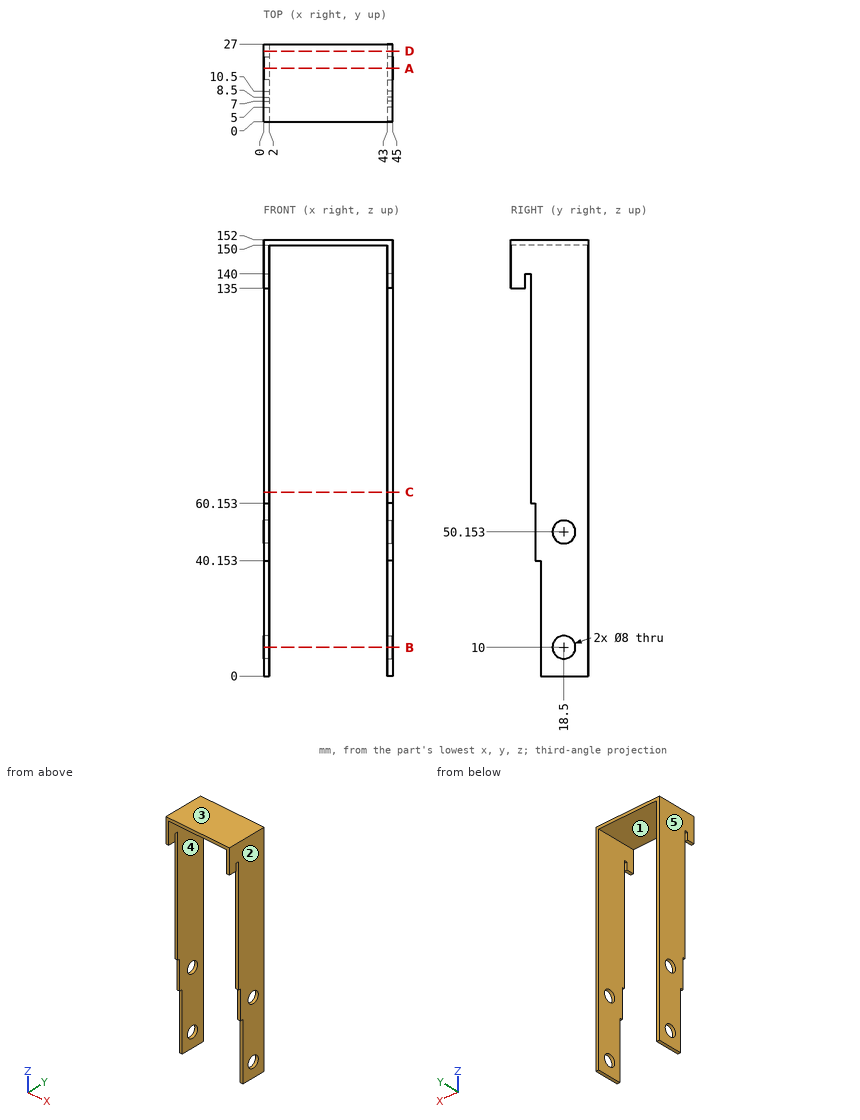
Source: three-view drawing plus pictorial views. Frame: mm from the lowest corner of the part. A direction names the side the tool comes from. Round coordinates to 2 decimals unless told otherwise and drop trailing zeros. Loops run counter-clockwise (first coordinate to the right, second up) from the corner with the lowest first, then second, coordinate; pieces in that order, holes last. Notation, with made-up numbers: (-7, -33) - (-2, -33) arc R25 cw to (-2, -19) - close; hole circle Ø8 at (77.25, 22.25). An arc over 180 degrees is marked (long way). Write item = value, one per line. Start each with the question number.
Item 1: Reachability of the marked faces 4 and 5 from +Z, -Z, +X, -X, +Y, -Y: full face, straight path, thin tool, end or side. Return the list, or none.
Item 2: First-contact query: pin 1 Ø1.5 at (y, z) = (8, 103.5) entering from -X; pin 2 Ø0.6 at (x, y) = (1, 10) entering from -Z; pin 3 Ø0.6 at (x, y) = (44, 1.5) entering from -Z; pin 4 Ø3 at (x, y) = (17, 19.5) entering from -Z. Flat tips, straight axial feed; report the tip coordinate or a pass-through.
Item 3: Mould query, pull axis X, two halves, no side actions, for the marked faces 1, 2 and 3. Classes: released by +X, released by -X, zero draft, split by the parting line, or undercut.
Item 4: Material intervals for line 1 (Z direction, x = 0.5, y = 18.5); line 2 (X direction, y = 23, z = 145); line 3 (Z direction, x = 29, y = 16.5), sorted ascending.
Item 5: Section query D-D on y = 24.5. Output: boundary loops of the cut face in (x, z).
Item 6: Section query B-B on z = 10. Output: boundary loops of the cut face in (x, y).
Item 7: Section query C-C on z = 64. Output: boundary loops of the cut face in (x, y).
Item 8: Section query A-A on y = 18.5. Output: boundary loops of the cut face in (x, z), plus the area to 3 significant figures.
Results list:
q1.face_4 = -Z, +Y, -Y
q1.face_5 = +Z, -Z, -X, +Y, -Y
q2.pin_1 = 0
q2.pin_2 = 40.15
q2.pin_3 = 135
q2.pin_4 = 150
q3.face_1 = undercut
q3.face_2 = released by +X
q3.face_3 = zero draft
q4.line_1 = 0 to 6, 14 to 46.15, 54.15 to 152
q4.line_2 = 0 to 2, 43 to 45
q4.line_3 = 150 to 152
q5.outline = (0, 0) - (2, 0) - (2, 150) - (43, 150) - (43, 0) - (45, 0) - (45, 152) - (0, 152) - close
q6.outline = (0, 10.5) - (2, 10.5) - (2, 14.5) - (0, 14.5) - close; (0, 22.5) - (2, 22.5) - (2, 27) - (0, 27) - close; (43, 10.5) - (45, 10.5) - (45, 14.5) - (43, 14.5) - close; (43, 22.5) - (45, 22.5) - (45, 27) - (43, 27) - close
q7.outline = (0, 7) - (2, 7) - (2, 27) - (0, 27) - close; (43, 7) - (45, 7) - (45, 27) - (43, 27) - close
q8.outline = (0, 0) - (2, 0) - (2, 6) - (0, 6) - close; (0, 14) - (2, 14) - (2, 46.15) - (0, 46.15) - close; (0, 54.15) - (2, 54.15) - (2, 150) - (43, 150) - (43, 54.15) - (45, 54.15) - (45, 152) - (0, 152) - close; (43, 0) - (45, 0) - (45, 6) - (43, 6) - close; (43, 14) - (45, 14) - (45, 46.15) - (43, 46.15) - close
q8.area = 626 mm²
